```python
from build123d import *

# Parameters (mm, degrees)
BOSS_EXTRUDE1_DEPTH     = 64
BOSS_EXTRUDE2_DEPTH     = 40
BOSS_EXTRUDE3_DEPTH     = 12
FILLET2_R               = 32
CUT_EXTRUDE1_DEPTH      = 125.963994815
CUT_EXTRUDE1_DEPTH_BACK = 125.963994815


with BuildPart() as part:
    # Sketch1 → Boss-Extrude1 (new body)
    with BuildSketch(Plane.XY):
        Polygon((96, 0), (96, 16), (16, 16), (16, 64), (0, 64), (0, 0), align=None)
    extrude(amount=BOSS_EXTRUDE1_DEPTH)

    # Sketch1_3 → Boss-Extrude2 (add)
    with BuildSketch(Plane.XY):
        with BuildLine():
            Line((24, 48), (16, 48))
            Line((16, 48), (16, 16))
            Line((16, 16), (56, 16))
            Line((56, 16), (56, 48))
            Line((56, 48), (48, 48))
            ThreePointArc((48, 48), (36, 36), (24, 48))
        make_face()
    extrude(amount=BOSS_EXTRUDE2_DEPTH)

    # Sketch1_4 → Boss-Extrude3 (add)
    with BuildSketch(Plane.XY):
        Polygon((56, 48), (56, 16), (96, 16), align=None)
    extrude(amount=BOSS_EXTRUDE3_DEPTH)

    # Fillet2
    fillet2_edges = [part.edges().sort_by_distance(p)[0] for p in [
        (8, 64, 64),
    ]]
    fillet(fillet2_edges, radius=FILLET2_R)

    # Sketch2 → Cut-Extrude1 (cut, two sides: drawn at the far end of the back side and taken through both)
    with BuildSketch(Plane(origin=(0, 16, 0), x_dir=(1, 0, 0), z_dir=(0, 1, 0)).offset(-CUT_EXTRUDE1_DEPTH_BACK)):
        with BuildLine():
            Line((96, -33.01098071), (76, -33.01098071))
            ThreePointArc((76, -33.01098071), (69.01098071, -40), (76, -46.98901929))
            Line((76, -46.98901929), (96, -46.98901929))
            Line((96, -46.98901929), (96, -33.01098071))
        make_face()
    extrude(amount=CUT_EXTRUDE1_DEPTH + CUT_EXTRUDE1_DEPTH_BACK, mode=Mode.SUBTRACT)


solid = part.part
```
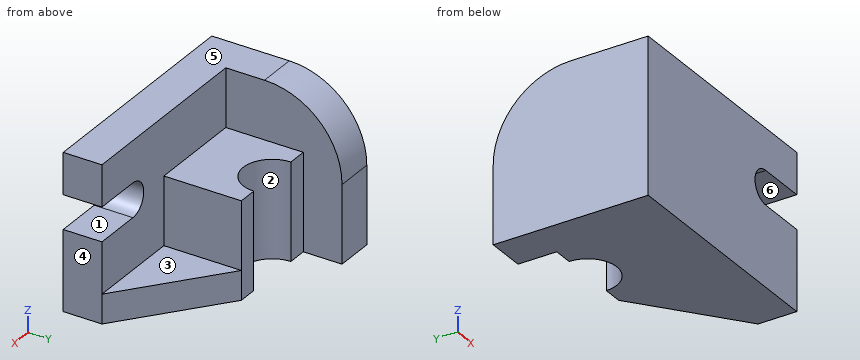
Geometry check sheet. Reference: the model listing, model coordinates, mm. Face numbers are marked on the shaded views. A direction names the side the tool comes from. Give positions to 0.01 mm unless a question says otherwise; leave off trailing zeros. Order: outer loops, then holes, each group sorted by start corner. A loop starts at its lowest first (then second) coordinate and runs counter-clockwise, first axis right, second up. Notation, with made-up numbers: (-26, 71) - (-11, 71) arc R25 ccw to (-11, 88) - close; hole circle Ø6 at (24, -40). An arc over 180 degrees is marked (long way). Answer in a Markdown table with one row per item. Add a question column.
Q1. Cross-section at B-B, the plane z = 30. Enter the section's corners in (x, y), then the cut area to 3 significant figures.
Q2. Mould release check, pull along Z, two halves, no side actions. Record for the marked faces 4, 5 and 6: pulls with the +Z half, pulls with the -Z half, needs draft (parallel to the pull), parting line crosses it, or undercut.
Q3. Cross-section at D-D, the plane y = 43.5. Enter the section's corners in (x, z) (3 decimals).
Q4. Tool access check on the marked faces 1, 2 and 3. Record the directions out of +Z, -Z, +X, -X, +Y, -Y that give a thin tool (end or side, any length) a straight path to the whole face; none if there is none.
Q5. Gauge pin test, flat ends, axial feed: pin 1 (12 mm diameter, centred on x = 45.5, z = 8, fed in from -Y); pin 2 (2 mm diameter, centred on x = 77, z = 13.5, fed in from +Y); pin 3 (12 mm diameter, centred on x = 66.5, y = 38, fed in from +Z); pin 4 (15.5 mm diameter, centred on x = 42, z = 38, fed in from +Y). Record the tip position at first contact, or that the pin passes through.
Q6. Cross-section at C-C, the plane x = 64. Enter the section's corners in (y, z), then the cut area to 3 significant figures.
Q7. Material ranges on probe 1 along Y at (x, z) = (23, 19.5); probe 2 along Z at (x, y) = (34, 30); probe 3 along Z at (x, y) = (71, 12), recorded low to high. Write a range as from..to.
Q8. Cross-section at A-A, the plane x = 87. Enter the section's corners in (y, z).
Check values:
| question | item | result |
|---|---|---|
| 1 | outline | (0, 0) - (96, 0) - (96, 16) - (56, 16) - (56, 48) - (48, 48) arc R12 cw to (24, 48) - (16, 48) - (16, 64) - (0, 64) - close |
| 1 | area | 3,360 mm^2 |
| 2 | face 4 | needs draft |
| 2 | face 5 | pulls with the +Z half |
| 2 | face 6 | undercut |
| 3 | outline | (0, 0) - (24.876, 0) - (24.876, 40) - (16, 40) - (16, 61.862) - (0, 61.862) - close; (47.124, 0) - (61.625, 0) - (61.625, 12) - (56, 12) - (56, 40) - (47.124, 40) - close |
| 4 | face 1 | +X, +Y, -Y |
| 4 | face 2 | +Z, -Z, +Y |
| 4 | face 3 | +Z, +X, +Y |
| 5 | pin 1 | stops at y = 0 |
| 5 | pin 2 | stops at y = 16 |
| 5 | pin 3 | stops at z = 12 |
| 5 | pin 4 | stops at y = 48 |
| 6 | outline | (0, 0) - (41.6, 0) - (41.6, 12) - (16, 12) - (16, 64) - (0, 64) - close |
| 6 | area | 1,330 mm^2 |
| 7 | probe 1 | y = 0..48 |
| 7 | probe 2 | z = 0..40 |
| 7 | probe 3 | z = 0..35.12, 44.88..64 |
| 8 | outline | (0, 0) - (23.2, 0) - (23.2, 12) - (16, 12) - (16, 33.01) - (0, 33.01) - close; (0, 46.99) - (16, 46.99) - (16, 64) - (0, 64) - close |
